The listing builds one solid part. Answer for the finished solid, in the listing's coordinates (mm). Face numbers are marked on the shaded views. Round coordinates to 2 decimals unless told otherwise and drop trailing zeros. Write each loop counter-clockwise with the first axis right and the second up, starting at its lowest first coordinate (ties: lowest second). Pieces come first, ordered by that corner, then holes.
Item 1: For a pull along Y with two mould halves and no side action, classify the marked faces 1, 2, 3 and 4 as +Y half, -Y half, draft (parallel to the pull), parting line (faces both ways), or undercut.
Item 2: Find section A-A on y = 0. Give the vertices of the cut face in (x, z), then the cut area to 3 significant figures.
Item 3: Find the intervals of material crossed by probe 1 along Y at (x, z) = (-18, 4.4); probe 2 along Y at (x, z) = (0, 3.45); probe 3 along Y at (x, z) = (0, -0.15), in increasing order.
Item 4: Find section B-B on x = 0. Give the vertices of the cut face in (y, z).
Item 5: Each of these flat-tipped pins is pushed along its axis until it touches: pin 1 (8 mm diameter, centred on x = 2.5, y = 30.5, fed in from +Z); pin 2 (22 mm diameter, centred on x = 3.5, y = 17, fed in from -Z); pin 3 (1.6 mm diameter, centred on x = -28.5, z = 4.5, fed in from -Y). Where does it stop, or does it pass through?
```python
from build123d import *

# Parameters (mm, degrees)
SKETCH_1_R               = 37
EXTRUDE_1_DEPTH          = 5
SKETCH_4_R               = 34.4
SKETCH_4_R_2             = 30.4
EXTRUDE_2_DEPTH          = 0.8
SKETCH_5_R               = 5.1
CUT_EXTRUDE_1_DEPTH      = 69.066144301
SKETCH_6_R               = 37
SKETCH_6_R_2             = 10
CUT_EXTRUDE_2_DEPTH      = 2
CUT_EXTRUDE_2_DRAFT      = -45
SKETCH_7_W               = 25.320983541
SKETCH_7_H               = 4
EXTRUDE_3_DEPTH          = 2
SKETCH_9_W               = 2
SKETCH_9_H               = 4
EXTRUDE_5_DEPTH          = 5
PATTERN_CIRCULAR_1_COUNT = 2


with BuildPart() as part:
    # 스케치1 → 보스-돌출1 (new body)
    with BuildSketch(Plane.XY):
        Circle(SKETCH_1_R)
    extrude(amount=EXTRUDE_1_DEPTH)

    # 스케치3 → 회전1 (revolve)
    with BuildSketch(Plane(origin=(0, 0, 0), x_dir=(1, 0, 0), z_dir=(0, 1, 0)), mode=Mode.PRIVATE) as revolve_1_sk:
        Polygon((-37, -5), (-37, 0), (-48, -5), align=None)
    revolve(revolve_1_sk.sketch.rotate(Axis((0, 0, -6.462572401), (0, 0, 1)), 180), axis=Axis((0, 0, -6.462572401), (0, 0, 1)))

    # 스케치4 → 보스-돌출2 (add)
    with BuildSketch(Plane(origin=(0, 0, 0), x_dir=(-1, 0, 0), z_dir=(0, 0, -1))):
        with Locations(Location((0, 0, 0), (0, 0, 180))):
            Circle(SKETCH_4_R)
        Circle(SKETCH_4_R_2, mode=Mode.SUBTRACT)
    extrude(amount=EXTRUDE_2_DEPTH)

    # 스케치5 → 컷-돌출1 (cut, through all)
    with BuildSketch(Plane(origin=(0, 0, 0), x_dir=(-1, 0, 0), z_dir=(0, 0, -1))):
        Circle(SKETCH_5_R)
    extrude(amount=-CUT_EXTRUDE_1_DEPTH, mode=Mode.SUBTRACT)


with BuildPart() as cut_extrude_2_tool:
    # 스케치6 → 컷-돌출2 (with draft: the straight prism first)
    with BuildSketch(Plane.XY.offset(5)):
        with Locations((0, 0.990500037)):
            Circle(SKETCH_6_R)
        Circle(SKETCH_6_R_2, mode=Mode.SUBTRACT)
    extrude(amount=-CUT_EXTRUDE_2_DEPTH)
    # 컷-돌출2: the draft: its side faces are tilted about the plane it starts from
    cut_extrude_2_sides = [cut_extrude_2_tool.faces().sort_by_distance(p)[0] for p in [
        (-37, 0.990500037, 4),
        (-10, 0, 4),
    ]]
    draft(cut_extrude_2_sides, Plane.XY.offset(5), CUT_EXTRUDE_2_DRAFT)


with BuildPart() as part_1:
    add(part.part)

    # 컷-돌출2: cut by cut_extrude_2_tool
    add(cut_extrude_2_tool.part, mode=Mode.SUBTRACT)

    # 스케치7 → 보스-돌출3 (add)
    with BuildSketch(Plane.XY.offset(5)):
        with Locations((-27.526560518, 0)):
            Rectangle(SKETCH_7_W, SKETCH_7_H)
    extrude_3 = extrude(amount=-EXTRUDE_3_DEPTH)

    # 스케치9 → 보스-돌출5 (add)
    with BuildSketch(Plane(origin=(-14.866068747, 0, 0), x_dir=(0, 0, -1), z_dir=(1, 0, 0))):
        with Locations((-4, 0)):
            Rectangle(SKETCH_9_W, SKETCH_9_H)
    extrude_5 = extrude(amount=EXTRUDE_5_DEPTH)

    # 원형 패턴1: 보스-돌출3, 보스-돌출5 ×2 about axis
    pattern_circular_1_axis = Axis((0, 0, 0), (0, 0, 1))
    add([extrude_3.rotate(pattern_circular_1_axis, i * 360 / PATTERN_CIRCULAR_1_COUNT) for i in range(1, PATTERN_CIRCULAR_1_COUNT)])
    add([extrude_5.rotate(pattern_circular_1_axis, i * 360 / PATTERN_CIRCULAR_1_COUNT) for i in range(1, PATTERN_CIRCULAR_1_COUNT)])


solid = part_1.part
```
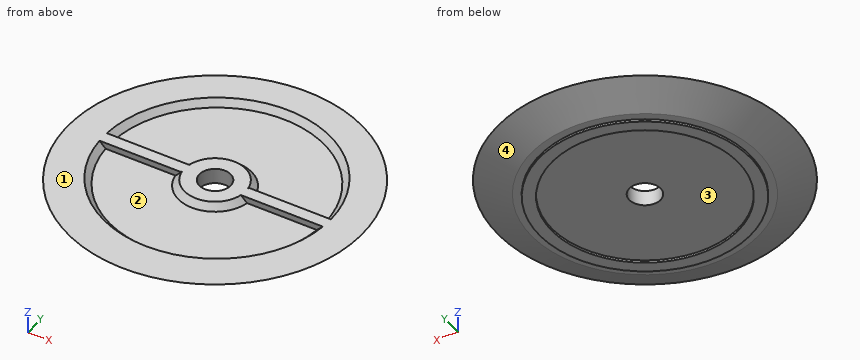
Check values:
1. face 1: draft
1. face 2: undercut
1. face 3: undercut
1. face 4: parting line
2. outline: (-48, 5) - (-37, 0) - (-34.4, 0) - (-34.4, -0.8) - (-30.4, -0.8) - (-30.4, 0) - (-5.1, 0) - (-5.1, 5) - close; (5.1, 0) - (30.4, 0) - (30.4, -0.8) - (34.4, -0.8) - (34.4, 0) - (37, 0) - (48, 5) - (5.1, 5) - close
2. area: 380 mm2
3. probe 1: y = -43.07 to -30.65, -2 to 2, 32.63 to 43.07
3. probe 2: y = -44.59 to -34.46, -11.55 to -5.1, 5.1 to 11.55, 36.44 to 44.59
3. probe 3: y = -34.4 to -30.4, 30.4 to 34.4
4. outline: (-48, 5) - (-37, 0) - (-34.4, 0) - (-34.4, -0.8) - (-30.4, -0.8) - (-30.4, 0) - (-5.1, 0) - (-5.1, 5) - (-10, 5) - (-12, 3) - (-34.01, 3) - (-36.01, 5) - close; (5.1, 0) - (30.4, 0) - (30.4, -0.8) - (34.4, -0.8) - (34.4, 0) - (37, 0) - (48, 5) - (37.99, 5) - (35.99, 3) - (12, 3) - (10, 5) - (5.1, 5) - close
5. pin 1: stops at z = 3
5. pin 2: stops at z = 0
5. pin 3: stops at y = -39.08
